Study the drawing (mm; zero at the part's minimum x, y, z) and answer. Coordinates: 2 decimals unless noted, no trailing zeros. Write each loop counter-clockwise with the first axis right and the second up, starting at its lowest first coordinate (ties: lowest second). Pieces come first, ordered by that corner, then holes. Notation, with made-up numbers: (-37, 9.5) -> (14, 9.5) arc R26 ccw to (14, 44.5) -> close; hole circle Ø11 at (-14, -6). An arc over 180 degrees is marked (long way). Answer in a Markdown table with one row per item. Add a question column.
Item 1: Section A-A on y = 21 is taken. Write down the section's boundary in (x, z).
Item 2: Section B-B on x = 21 is taken. Write down the section's boundary in (y, z), then the cut area to 3 significant figures.
Item 3: Section C-C on x = 14 is taken. Write down the section's boundary in (y, z), then the cut area to 3 significant figures.
Item 4: Given pin 1 Ø1 at (y, z) = (45.5, 1) entering from -X; pin 2 Ø1 at (y, z) = (34, 1) entering from -X; pin 3 Ø10 at (x, y) = (25, 16) entering from -Z, each flat-ended and moving along its own axis, determine where each tip first touches the part or whether it passes through.
Item 5: Straight lines are drawn through the part: line 1 (Y direction, x = 21, z = 0.5); line 2 (X direction, y = 32.5, z = 0.55); line 3 (X direction, y = 48.5, z = 0.75). For each, find the intervals that lie inside material, in ascending order. Write a range as from..to.
Item 6: Section D-D on z = 0.9 is taken. Write down the section's boundary in (x, y), then the cut area to 3 significant figures.
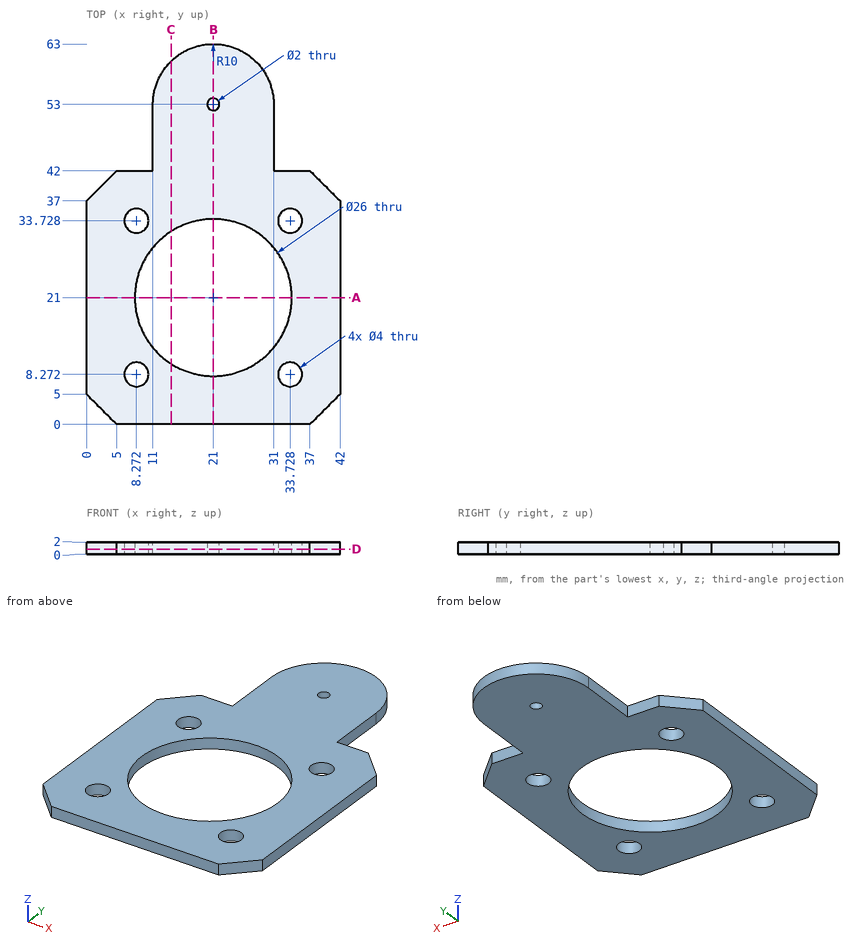
Results below:
| question | item | result |
|---|---|---|
| 1 | outline | (0, 0) -> (8, 0) -> (8, 2) -> (0, 2) -> close; (34, 0) -> (42, 0) -> (42, 2) -> (34, 2) -> close |
| 2 | outline | (0, 0) -> (8, 0) -> (8, 2) -> (0, 2) -> close; (34, 0) -> (52, 0) -> (52, 2) -> (34, 2) -> close; (54, 0) -> (63, 0) -> (63, 2) -> (54, 2) -> close |
| 2 | area | 70.0 mm2 |
| 3 | outline | (0, 0) -> (10.05, 0) -> (10.05, 2) -> (0, 2) -> close; (31.95, 0) -> (60.14, 0) -> (60.14, 2) -> (31.95, 2) -> close |
| 3 | area | 76.5 mm2 |
| 4 | pin 1 | stops at x = 11 |
| 4 | pin 2 | stops at x = 0 |
| 4 | pin 3 | passes through |
| 5 | line 1 | y = 0..8, 34..52, 54..63 |
| 5 | line 2 | x = 0..6.69, 9.85..14.94, 27.06..32.15, 35.31..42 |
| 5 | line 3 | x = 11..31 |
| 6 | outline | (0, 5) -> (5, 0) -> (37, 0) -> (42, 5) -> (42, 37) -> (37, 42) -> (31, 42) -> (31, 53) arc R10 ccw to (11, 53) -> (11, 42) -> (5, 42) -> (0, 37) -> close; hole circle Ø4 at (8.27, 8.27); hole circle Ø4 at (8.27, 33.73); hole circle Ø26 at (21, 21); hole circle Ø2 at (21, 53); hole circle Ø4 at (33.73, 8.27); hole circle Ø4 at (33.73, 33.73) |
| 6 | area | 1,510 mm2 |
